Can you work these out from the drawing? Everything is in mm from the part's minimum corner. A direction names the side the tool comes from. Give positions to 0.01 mm unless a question says otherwise; leave off trailing zeros. Loops run counter-clockwise (first coordinate to the right, second up) from the corner with the lowest first, then second, coordinate; pieces in that order, holes last. Notation, with made-up numbers: (-10.5, 12.25) - (28.5, 12.25) arc R17 ccw to (28.5, 38.25) - close; hole circle Ø1 at (-18, -31). An arc over 180 degrees is marked (long way). Answer in a Markdown table with one row per item.
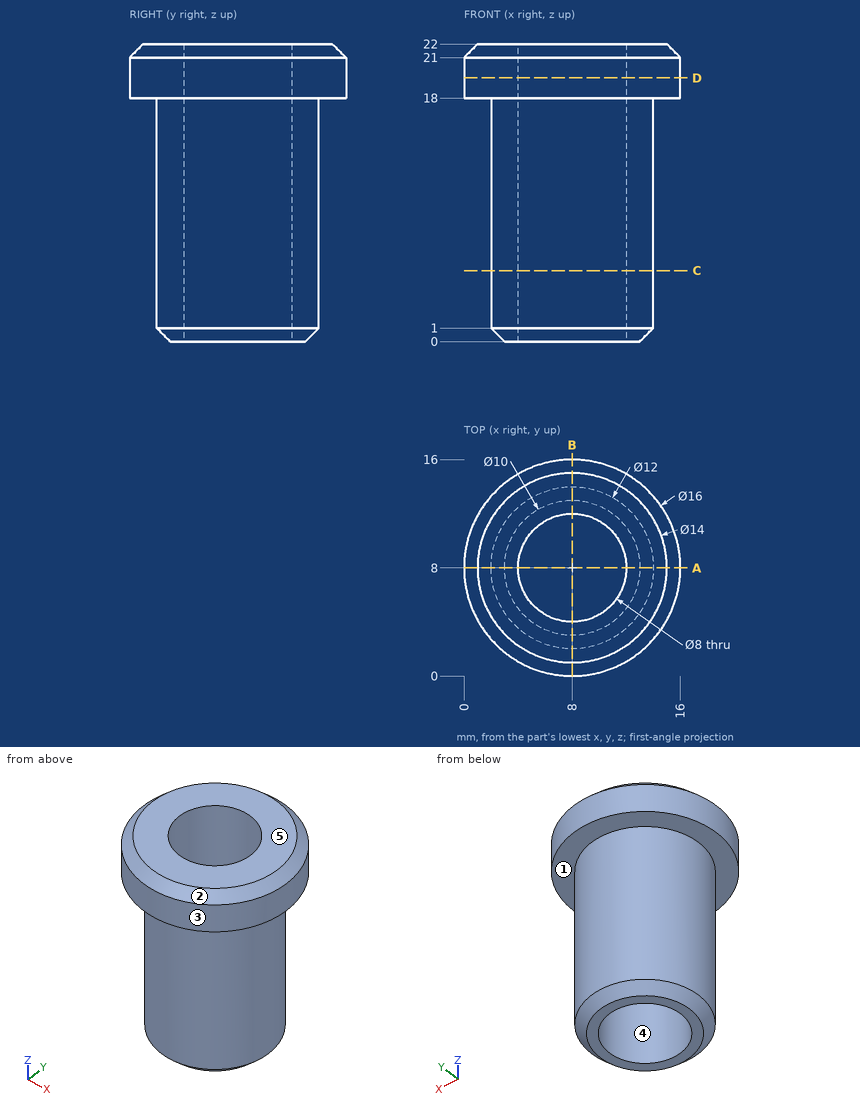
Q1. Imagine slicing it at A-A, the plane y = 8. Write out the boundary of the cut face in (x, z).
Checked values:
| item | result |
|---|---|
| outline | (0, 18) - (2, 18) - (2, 1) - (3, 0) - (4, 0) - (4, 22) - (1, 22) - (0, 21) - close; (12, 0) - (13, 0) - (14, 1) - (14, 18) - (16, 18) - (16, 21) - (15, 22) - (12, 22) - close |
Q2. If I drill on line 1 (Y direction, x = 8, z = 20); line 2 (Y direction, x = 8, z = 8.5); line 3 (X direction, y = 9, z = 14.25), over which ranges is the centre line in solid material (lowest first)? Write a range as [from, to].
Checked values:
| item | result |
|---|---|
| line 1 | y = [0, 4], [12, 16] |
| line 2 | y = [2, 4], [12, 14] |
| line 3 | x = [2.08, 4.13], [11.87, 13.92] |
Q3. If we mould it in two halves opening along Y, with no side actions, what happens to the marked faces 3, 4 and 5? For each: released by +Y, released by -Y, zero draft, split by the parting line, or undercut.
Checked values:
| item | result |
|---|---|
| face 3 | split by the parting line |
| face 4 | undercut |
| face 5 | zero draft |
Q4. For pin 1 (5 mm diameter, centred on y = 5.5, z = 6, fed in from +X); pin 2 (8 mm diameter, centred on x = 3, z = 3, fed in from +Y); pin 3 (3 mm diameter, centred on x = 12.5, z = 7, fed in from -Y), each with a flat end and sliding along its axis, tell me the tip position at first contact or that it passes through.
Checked values:
| item | result |
|---|---|
| pin 1 | stops at x = 14 |
| pin 2 | stops at y = 13.92 |
| pin 3 | stops at y = 2.8 |
Q5. Imagine slicing it at C-C, the plane z = 5.25. Write out the boundary of the cut face in (x, y).
Checked values:
| item | result |
|---|---|
| outline | circle Ø12 at (8, 8); hole circle Ø8 at (8, 8) |
Q6. Imagine slicing it at D-D, the plane z = 19.5. Write out the boundary of the cut face in (x, y), and give its area (3 significant figures).
Checked values:
| item | result |
|---|---|
| outline | circle Ø16 at (8, 8); hole circle Ø8 at (8, 8) |
| area | 151 mm² |
Q7. On a 3-axis mill with a long thin cutter (end or side, diameter ignored), from which of +Z, -Z, +X, -X, +Y, -Y can I reach the whole of each face in a straight line? I mean the marked faces 1 and 2. Say none if no direction works.
Checked values:
| item | result |
|---|---|
| face 1 | -Z |
| face 2 | +Z |
